from build123d import *

# Parameters (mm, degrees)
SKETCH5_W               = 127
SKETCH5_H               = 127
SKETCH5_R               = 38.1
SKETCH5_R_2             = 3.175
BOSS_EXTRUDE2_DEPTH     = 17.50822
SKETCH4_R               = 1.03251
CUT_EXTRUDE3_DEPTH      = 3.175
CIRPATTERN1_COUNT       = 9
CUT_EXTRUDE5_REACH      = 145.066
SKETCH8_R               = 3.175
CUT_EXTRUDE9_REACH      = 165.579
CUT_EXTRUDE9_END_RADIUS = 3.175
SKETCH10_R              = 0.79375


with BuildPart() as part:
    # Sketch1 → Revolve1 (revolve)
    with BuildSketch(Plane.XY, mode=Mode.PRIVATE) as revolve1_sk:
        with BuildLine():
            Line((-32.14624, 17.50822), (0, 17.50822))
            Line((0, 17.50822), (0, 0))
            Line((0, 0), (-27.1145, 0))
            Line((-27.1145, 0), (-27.1145, 3.456354569))
            ThreePointArc((-27.1145, 3.456354569), (-27.522854569, 4.980354569), (-28.6385, 6.096))
            Line((-28.6385, 6.096), (-32.14624, 8.96874))
            Line((-32.14624, 8.96874), (-32.14624, 17.50822))
        make_face()
    revolve(revolve1_sk.sketch.rotate(Axis((-38.1, 101.60464546, 0), (0, 1, 0)), 90), axis=Axis((-38.1, 101.60464546, 0), (0, 1, 0)))

    # Sketch5 → Boss-Extrude2 (add)
    with BuildSketch(Plane.XZ):
        with Locations((-38.1, 0)):
            Rectangle(SKETCH5_W, SKETCH5_H)
        with Locations((-38.1, 0)):
            Circle(SKETCH5_R, mode=Mode.SUBTRACT)
        with Locations(Location((-95.25, 57.15, 0), (0, 0, 270))):
            Circle(SKETCH5_R_2, mode=Mode.SUBTRACT)
        with Locations(Location((19.05, 57.15, 0), (0, 0, 90))):
            Circle(SKETCH5_R_2, mode=Mode.SUBTRACT)
        with Locations(Location((19.05, -57.15, 0), (0, 0, 270))):
            Circle(SKETCH5_R_2, mode=Mode.SUBTRACT)
        with Locations(Location((-95.25, -57.15, 0), (0, 0, 90))):
            Circle(SKETCH5_R_2, mode=Mode.SUBTRACT)
    extrude(amount=-BOSS_EXTRUDE2_DEPTH)

    # Sketch4 → Cut-Extrude3 (cut)
    with BuildSketch(Plane(origin=(0, 0, 0), x_dir=(-1, 0, 0), z_dir=(0, -1, 0))):
        with Locations(Location((82.55, 0, 0), (0, 0, 90))):
            Circle(SKETCH4_R)
    cut_extrude3 = extrude(amount=-CUT_EXTRUDE3_DEPTH, mode=Mode.SUBTRACT)

    # CirPattern1: Cut-Extrude3 ×9 about axis
    cirpattern1_axis = Axis((-38.1, 0, 0), (0, 1, 0))
    for i in range(1, CIRPATTERN1_COUNT):
        add(cut_extrude3.rotate(cirpattern1_axis, i * 360 / CIRPATTERN1_COUNT), mode=Mode.SUBTRACT)

    # Sketch8 → Cut-Extrude5 (cut, up to next)
    with BuildSketch(Plane(origin=(25.4, 0, 0), x_dir=(0, 0, -1), z_dir=(1, 0, 0)), mode=Mode.PRIVATE) as cut_extrude5_sk1:
        with Locations((0, 5.588)):
            Circle(SKETCH8_R)
    cut_extrude5_tool1 = extrude(cut_extrude5_sk1.sketch, amount=-CUT_EXTRUDE5_REACH, mode=Mode.PRIVATE) & part.part
    add(cut_extrude5_tool1.solids().sort_by_distance((25.4, 5.588, 0))[0], mode=Mode.SUBTRACT)

    # Cut-Extrude9: up to this cylinder (the profile starts outside it)
    cut_extrude9_end = Plane(origin=(-6.35, 5.588, 0), z_dir=(1, 0, 0)) * Cylinder(CUT_EXTRUDE9_END_RADIUS, 338.508, mode=Mode.PRIVATE)
    # Sketch10 → Cut-Extrude9 (cut, up to the surface)
    with BuildSketch(Plane.XY.offset(63.5), mode=Mode.PRIVATE) as cut_extrude9_sk1:
        with Locations((-6.35, 5.588)):
            Circle(SKETCH10_R)
    cut_extrude9_tool1 = extrude(cut_extrude9_sk1.sketch, amount=-CUT_EXTRUDE9_REACH, mode=Mode.PRIVATE) - cut_extrude9_end
    add(cut_extrude9_tool1.solids().sort_by_distance((-6.35, 5.588, 63.5))[0], mode=Mode.SUBTRACT)


solid = part.part
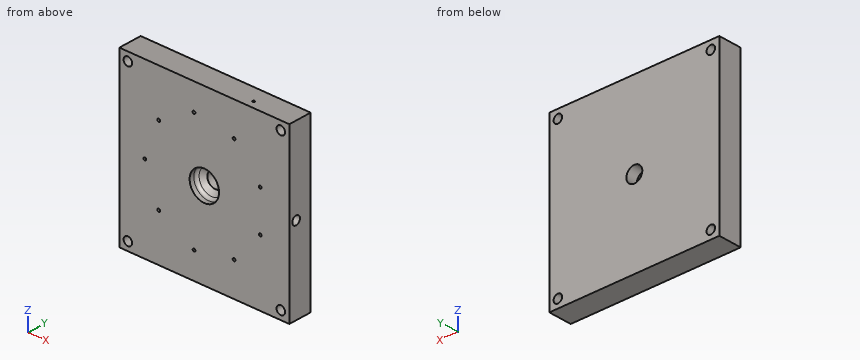
Check sheet for the modelled part. Datum: model origin and axes. Units: mm. Give positions to 0.01 mm unless a question says otherwise; leave off trailing zeros. Write each loop counter-clockwise with the first axis right and the second up, starting at its lowest first coordinate (ties: lowest second). Pieces come first, ordered by that corner, then holes. Notation, with made-up numbers: M 46.25,88 L 69.25,88 A16 cw 69.25,102 Z; hole C -34,84 d7. An arc over 180 degrees is marked long. Use one line per item in the form item = value.
(1) Depth check by flat-ended pin: P1, Ø1.9, axis at x = -72.15, z = -28.57, coming from the -Y side (3 decimals); P2, Ø4, axis at x = -65.5, z = 36, coming from the -Y side. Enter the tip coordinate at first touch or a pass-through.
Answer block:
P1 = 3.175
P2 = 0
(2) Section check B-B on z = 57.15. State how many separate pieces and enclosed holes the cut face has, plus the area to 3 significant figures.
Answer block:
separate_pieces = 3
enclosed_holes = 1
area = 2,000 mm2
(3) Section check A-A on x = 19.05. Record the boundary of the cut face in (y, z) (3 decimals), plus the area to 3 significant figures.
Answer block:
outline = M 0,-63.5 L 17.508,-63.5 L 17.508,-60.325 L 0,-60.325 Z; M 0,-53.975 L 17.508,-53.975 L 17.508,53.975 L 0,53.975 Z; M 0,60.325 L 17.508,60.325 L 17.508,63.5 L 0,63.5 Z; hole C 5.588,0 d6.35
area = 1,970 mm2
(4) Section check C-C on z = -57.15. Record the boundary of the cut face in (x, y) (3 decimals).
Answer block:
outline = M -101.6,0 L -98.425,0 L -98.425,17.508 L -101.6,17.508 Z; M -92.075,0 L 15.875,0 L 15.875,17.508 L -92.075,17.508 Z; M 22.225,0 L 25.4,0 L 25.4,17.508 L 22.225,17.508 Z
(5) Material ranges on line 1 along Z through (x, y) = (19.5, 1.5); line 2 along X through (y, z) = (10.5, -57.15) (3 decimals); line 3 along X through (y, z) = (5.5, 41.5), recorded low to high.
Answer block:
line_1 = -63.5 to -60.29, -54.01 to 54.01, 60.29 to 63.5
line_2 = -101.6 to -98.425, -92.075 to 15.875, 22.225 to 25.4
line_3 = -101.6 to -7.14, -5.56 to 25.4
